Autodesk Inventor part; units mm, degrees
ref_plane "YZ Plane" through (0, 0, 0) normal (1, 0, 0) x (0, 1, 0)
ref_plane "XZ Plane" through (0, 0, 0) normal (0, 1, 0) x (-1, 0, 0)
ref_plane "XY Plane" through (0, 0, 0) normal (0, 0, 1) x (1, 0, 0)
sketch "Sketch1" plane through (0, 0, 0) normal (0, 1, 0) x (-1, 0, 0)
  line L0 (75, 37.5) -> (-75, 37.5)
  line L1 (-75, 37.5) -> (-75, -37.5)
  line L2 (-75, -37.5) -> (75, -37.5)
  line L3 (75, -37.5) -> (75, 37.5)
  point P0 (0, 0)
  dimension "d0" = 150
  dimension "d1" = 75
  dimension "d2" = 75
  dimension "d3" = 37.5
extrude "Extrusion1" add sketch "Sketch1" along normal blind 9
sketch "Sketch3" plane through (0, 9, 0) normal (0, 1, 0) x (1, 0, 0)
  line L0 (-75, -37.5) -> (75, -37.5)
  line L1 (75, -37.5) -> (75, 37.5)
  line L2 (75, 37.5) -> (-75, 37.5)
  line L3 (-75, 37.5) -> (-75, -37.5)
  circle A0 centre (-44, 0) radius 12
  point P0 (0, 0)
  dimension "d11" = 24
  dimension "d12" = 19
  dimension "d13" = 31
extrude "Extrusion3" add sketch "Sketch3" along normal blind 2 contours A0
properties part number "Phone"
Can you work these out from the model? Positions are in its coordinate system, mm. A direction names the side the tool comes from. Give positions to 0.01 mm unless a question says otherwise; leave off trailing zeros. Loops run counter-clockwise (first coordinate to the right, second up) from the corner with the lowest first, then second, coordinate; pieces in that order, holes last. Notation, with made-up numbers: (44, -39) -> (103, -39) arc R20 cw to (103, -2) -> close; hole circle Ø4 at (-15.75, 55). An arc over 180 degrees is marked (long way). Write item = value, one per line.
1) Suppose I cut it at B-B on x = -44. Write out the boundary of the cut face in (y, z), then the cut area to 3 significant figures.
Check result:
outline = (0, -37.5) -> (9, -37.5) -> (9, -12) -> (11, -12) -> (11, 12) -> (9, 12) -> (9, 37.5) -> (0, 37.5) -> close
area = 723 mm2
2) I need wall thicknesses on L1, parallel to Y at x = 42, z = 3; L2, parallel to Z at x = -54, y = 9.25; L3, parallel to X at y = 9.75, z = 10.5. Which ranges of each line are inside material? Lowest first, please. Write a range as from..to.
Check result:
L1 = 0..9
L2 = -6.63..6.63
L3 = -49.81..-38.19
3) Will this pin go through, and if not, where does the flat tip stop? pin 1 (10 mm diameter, centred on x = 43.5, z = -10, fed in from +Y).
Check result:
pin_1 = 9
4) Suppose I cut it at D-D on x = 24. Write out the boundary of the cut face in (y, z).
Check result:
outline = (0, -37.5) -> (9, -37.5) -> (9, 37.5) -> (0, 37.5) -> close
5) Suppose I cut it at A-A on z = 0. Write out the boundary of the cut face in (x, y).
Check result:
outline = (-75, 0) -> (75, 0) -> (75, 9) -> (-32, 9) -> (-32, 11) -> (-56, 11) -> (-56, 9) -> (-75, 9) -> close
6) For faces 1 (the flat face through (-44, 11, 0)), 2 (the cylindrical face through (-53.523, 9.986, -7.302)), which set-ups out of +Z, -Z, +X, -X, +Y, -Y let a thin tool reach every point of the face, with its end or its side?
Check result:
face_1 = +Z, -Z, +X, -X, +Y
face_2 = +Y
7) Suppose I cut it at C-C on z = -24. Write out the boundary of the cut face in (x, y).
Check result:
outline = (-75, 0) -> (75, 0) -> (75, 9) -> (-75, 9) -> close
